Build history of the part. All positions in model axes, mm. A direction names the side the tool comes from. Give positions to 0.01 mm unless a question says otherwise; leave off trailing zeros. Write each loop counter-clockwise with the first axis right and the second up, starting at its lowest first coordinate (ties: lowest second). Pieces come first, ordered by that corner, then holes. Notation, with made-up numbers: (14, -16) -> (46, -16) arc R19 cw to (46, 6) -> close; hole circle Ø1 at (59, 61.5). An arc over 180 degrees is marked (long way). One line per question, with ' | ' between items. Start each with the question number.
(1) Tool access for faces 1 (the flat face through (5, 150, 0)), 2 (the flat face through (0.508, 150, -5)): list every direction of +Z, -Z, +X, -X, +Y, -Y with a clear straight run to the whole face (end or side of a thin tool).
(2) Band-saw the part on A-A, the plane y = 151. Give the cut face in (x, z) (3 decimals), and give its area (3 significant figures).
(3) Pin check, flat tips, straight feed: P1, Ø2.5, axis at y = 148.5, z = -4.5, coming from the +X side; P2, Ø2.5, axis at x = 5.02, y = 222.25, coming from the -Z side; P3, Ø5, axis at x = 5.02, y = 171.45, coming from the -Z side. Stop position of each tip, or through.
(4) Drill centre lines: probe 1 along X at (y, z) = (273.05, -0.2) (3 decimals); probe 2 along Z at (x, y) = (2.5, 109); probe 3 along X at (y, z) = (14.5, -5.75). Where is each one in solid material? Low to high. Write a range as from..to.
from build123d import *

# Parameters (mm, degrees)
BOSS_EXTRUDE1_DEPTH = 304.8
SKETCH3_R           = 1.5875
CUT_EXTRUDE1_DEPTH  = 306.082074062
LPATTERN1_COUNT     = 12
LPATTERN1_PITCH     = 25.4
SKETCH4_R           = 1.5875
CUT_EXTRUDE2_DEPTH  = 306.082074062
LPATTERN2_COUNT     = 12
LPATTERN2_PITCH     = 25.4


with BuildPart() as part:
    # Sketch2 → Boss-Extrude1 (new body)
    with BuildSketch(Plane(origin=(0, 0, 0), x_dir=(1, 0, 0), z_dir=(0, 1, 0))):
        Polygon((0, 0), (9.525, 0), (9.525, 0.508), (0.508, 0.508), (0.508, 9.525), (0, 9.525), align=None)
    extrude(amount=BOSS_EXTRUDE1_DEPTH)

    # Sketch3 → Cut-Extrude1 (cut, through all)
    with BuildSketch(Plane(origin=(0, 0, -0.508), x_dir=(-1, 0, 0), z_dir=(0, 0, -1))):
        with Locations((-5.0165, 298.45)):
            Circle(SKETCH3_R)
    cut_extrude1 = extrude(amount=-CUT_EXTRUDE1_DEPTH, mode=Mode.SUBTRACT)

    # LPattern1: Cut-Extrude1 ×12
    with Locations(*[(0, -i * LPATTERN1_PITCH, 0) for i in range(1, LPATTERN1_COUNT)]):
        add(cut_extrude1, mode=Mode.SUBTRACT)

    # Sketch4 → Cut-Extrude2 (cut, through all)
    with BuildSketch(Plane(origin=(0.508, 0, 0), x_dir=(0, 0, -1), z_dir=(1, 0, 0))):
        with Locations((5.0165, 285.75)):
            Circle(SKETCH4_R)
    cut_extrude2 = extrude(amount=-CUT_EXTRUDE2_DEPTH, mode=Mode.SUBTRACT)

    # LPattern2: Cut-Extrude2 ×12
    with Locations(*[(0, -i * LPATTERN2_PITCH, 0) for i in range(1, LPATTERN2_COUNT)]):
        add(cut_extrude2, mode=Mode.SUBTRACT)


solid = part.part
Results:
1) face 1: +Z, +X, -X, +Y, -Y | face 2: -Z, +X, +Y, -Y
2) outline: (0, -9.525) -> (0.508, -9.525) -> (0.508, -0.508) -> (9.525, -0.508) -> (9.525, 0) -> (0, 0) -> close | area: 9.42 mm²
3) P1: stops at x = 0.51 | P2: passes through | P3: stops at z = -0.51
4) probe 1: x = 0..3.429, 6.604..9.525 | probe 2: z = -0.51..0 | probe 3: x = 0..0.51
